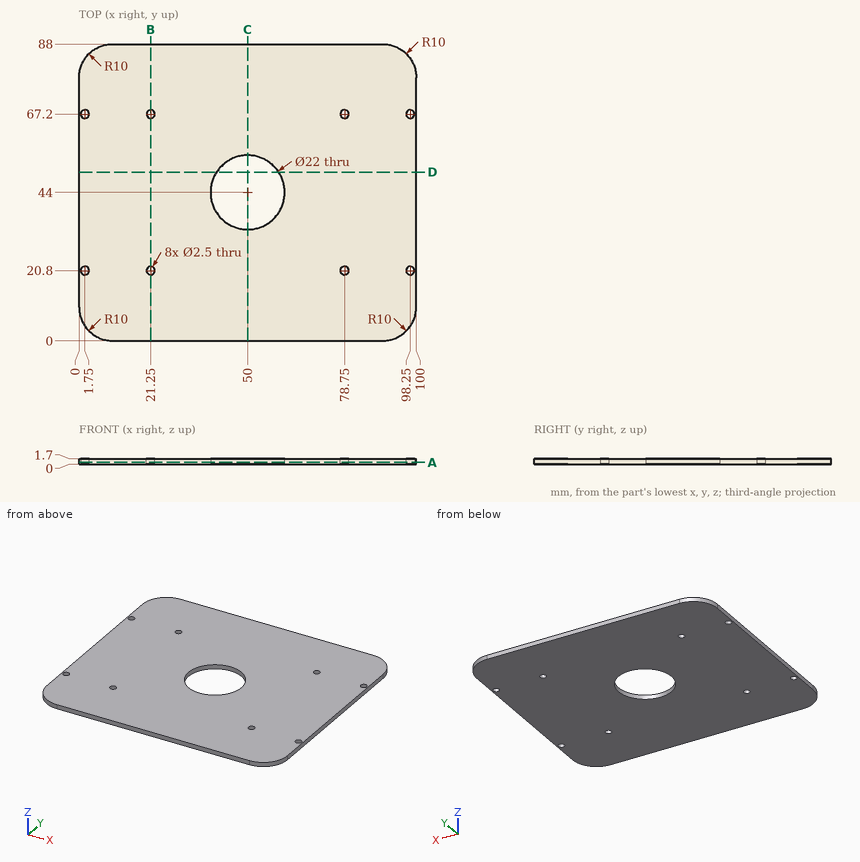
Source: three-view drawing plus pictorial views. Frame: mm from the lowest corner of the part. Give positions to 0.01 mm unless a question says otherwise; leave off trailing zeros. Write each loop counter-clockwise with the first axis right and the second up, starting at its lowest first coordinate (ties: lowest second). Pieces come first, ordered by that corner, then holes. Notation, with made-up numbers: M 61,-8 L 71,-8 A19 cw 71,7 Z; hole C -4.75,-31.5 d2. An arc over 180 degrees is marked long. Use one line per item in the form item = value.
1. Cut plane B-B on x = 21.25. Return loops of the section in (y, z), and give its area (3 significant figures).
Outcome:
outline = M 0,0 L 19.55,0 L 19.55,1.7 L 0,1.7 Z; M 22.05,0 L 65.95,0 L 65.95,1.7 L 22.05,1.7 Z; M 68.45,0 L 88,0 L 88,1.7 L 68.45,1.7 Z
area = 141 mm²
2. Ray query, L1, parallel to Y at x = 78.75, z = 1.35; L2, parallel to X at y = 67.2, z = 1; L3, parallel to Y at x = 98.25, z = 1.25. Return the intervals inside material, ascending.
Outcome:
L1 = 0 to 19.55, 22.05 to 65.95, 68.45 to 88
L2 = 0 to 0.5, 3 to 20, 22.5 to 77.5, 80 to 97, 99.5 to 100
L3 = 4.35 to 19.55, 22.05 to 65.95, 68.45 to 83.65
3. Cut plane A-A on z = 0.6. State how many separate pieces and enclosed holes the cut face has, and give its area (3 significant figures).
Outcome:
separate_pieces = 1
enclosed_holes = 9
area = 8,290 mm²
4. Cut plane D-D on y = 50. Return loops of the section in (x, z).
Outcome:
outline = M 0,0 L 40.78,0 L 40.78,1.7 L 0,1.7 Z; M 59.22,0 L 100,0 L 100,1.7 L 59.22,1.7 Z
5. First-contact query: P1, Ø1, axis at x = 73, z = 1, coming from the -Y side. Flat tip, straight axial feed; report the tip coordinate or a pass-through.
Outcome:
P1 = 0
6. Cut plane C-C on x = 50. Return loops of the section in (y, z).
Outcome:
outline = M 0,0 L 33,0 L 33,1.7 L 0,1.7 Z; M 55,0 L 88,0 L 88,1.7 L 55,1.7 Z
